```python
from build123d import *

# Parameters (mm, degrees)
F0_W     = 101.6
F0_H     = 50.8
F1_DEPTH = 25.4
F2_R     = 6.35
F3_DEPTH = 25.401
F5_W     = 7.62
F5_H     = 7.62
F6_ANGLE = 30


with BuildPart() as f1:
    # F0 (on Front) → F1 (new body)
    with BuildSketch(Plane.XZ):
        Rectangle(F0_W, F0_H)
    extrude(amount=-F1_DEPTH)

    # F2 (on face) → F3 (cut, through all)
    with BuildSketch(Plane.XZ):
        with Locations((-38.1, 12.7)):
            Circle(F2_R)
        with Locations((-38.1, -12.7)):
            Circle(F2_R)
        with Locations((38.1, 12.7)):
            Circle(F2_R)
        with Locations((38.1, -12.7)):
            Circle(F2_R)
    extrude(amount=-F3_DEPTH, mode=Mode.SUBTRACT)

    # F4 (on Top) + F5 (on Top) → F6 (revolve, cut)
    with BuildSketch(Plane.XY):
        Polygon((0, 25.4), (0, 50.8), (-12.7, 50.8), (-12.7, 25.4), (-10.645107, 25.4), (-6.35, 25.4), align=None)
    with BuildSketch(Plane.XY):
        with Locations((8.859598, 41.420042)):
            Rectangle(F5_W, F5_H)
    revolve(axis=Axis((0, 38.1, 0), (0, -1, 0)), revolution_arc=F6_ANGLE, mode=Mode.SUBTRACT)

    # F5 (on Top) → F7 (revolve, cut)
    with BuildSketch(Plane.XY):
        with Locations((8.859598, 41.420042)):
            Rectangle(F5_W, F5_H)
    revolve(axis=Axis((0, 38.1, 0), (0, -1, 0)), mode=Mode.SUBTRACT)


solid = f1.part
```
Design review of the part built by this model. Coordinates are the model's own, in mm. Round coordinates to 2 decimals unless told otherwise and drop trailing zeros. Write each loop counter-clockwise with the first axis right and the second up, starting at its lowest first coordinate (ties: lowest second). Pieces come first, ordered by that corner, then holes. Notation, with made-up numbers: (-12, -29.5) -> (-5, -29.5) arc R21 cw to (-5, -4.5) -> close; hole circle Ø10 at (43, 45). An arc over 180 degrees is marked (long way). Write item = value, one per line. Start each with the question number.
1) Mouldability with a two-part tool opening along X and no side actions: class faces 1 (the face through (-32.234, 12.522, -15.132)), 2 (the face through (-1, 0, 0)), 3 (the face through (-50.8, 13, 0)) as +X half, -X half, draft (parallel to the pull), parting line (faces both ways), or undercut.
2) Wall thickness on probe 1 along Z at (x, y) = (-38.1, 10); probe 2 along X at (y, z) = (10, 11); probe 3 along X at (y, z) = (5.75, -8): over which ranges is each line inside the solid? List them lowest first. Write a range as from..to.
3) Clearance check with a flat-ended pin moving along its axis: pin 1 (7.5 mm diameter, centred on x = 38.1, z = -12.7, fed in from +Y). State where the tip first meets the part, or that it passes through.
4) Take a section at A-A, the plane x = -38.1. State the section outline as (y, z) points, plus the area to 3 significant figures.
5) Take a section at C-C, the plane y = 16. State the section outline as (x, z) points, plus the area to 3 significant figures.
6) Take a section at B-B, the plane z = 12.7. State the section outline as (x, y) points, plus the area to 3 significant figures.
Results list:
q1.face_1 = undercut
q1.face_2 = draft
q1.face_3 = -X half
q2.probe_1 = -25.4..-19.05, -6.35..6.35, 19.05..25.4
q2.probe_2 = -50.8..-44.22, -31.98..31.98, 44.22..50.8
q2.probe_3 = -50.8..-42.37, -33.83..33.83, 42.37..50.8
q3.pin_1 = through
q4.outline = (0, -25.4) -> (25.4, -25.4) -> (25.4, -19.05) -> (0, -19.05) -> close; (0, -6.35) -> (25.4, -6.35) -> (25.4, 6.35) -> (0, 6.35) -> close; (0, 19.05) -> (25.4, 19.05) -> (25.4, 25.4) -> (0, 25.4) -> close
q4.area = 645 mm²
q5.outline = (-50.8, -25.4) -> (50.8, -25.4) -> (50.8, 25.4) -> (-50.8, 25.4) -> close; hole circle Ø12.7 at (-38.1, -12.7); hole circle Ø12.7 at (-38.1, 12.7); hole circle Ø12.7 at (38.1, -12.7); hole circle Ø12.7 at (38.1, 12.7)
q5.area = 4,650 mm²
q6.outline = (-50.8, 0) -> (-44.45, 0) -> (-44.45, 25.4) -> (-50.8, 25.4) -> close; (-31.75, 0) -> (31.75, 0) -> (31.75, 25.4) -> (-31.75, 25.4) -> close; (44.45, 0) -> (50.8, 0) -> (50.8, 25.4) -> (44.45, 25.4) -> close
q6.area = 1,940 mm²
